from build123d import *

# Parameters (mm, degrees)
F0_W      = 46
F0_H      = 40
F1_DEPTH  = 46
F2_R      = 9
F3_DEPTH  = 30
F4_R      = 9
F5_DEPTH  = 30
F6_W      = 24
F6_H      = 30
F7_DEPTH  = 46
F9_R      = 18
F10_DEPTH = 25
F8_R      = 9
F11_DEPTH = 30
F12_R     = 18
F13_DEPTH = 30
F14_R     = 9
F15_DEPTH = 30


with BuildPart() as f1:
    # F0 (on Top) → F1 (new body)
    with BuildSketch(Plane.XY):
        with Locations((-30.6679215729, -38.7895996869)):
            Rectangle(F0_W, F0_H)
    extrude(amount=F1_DEPTH)

    # F2 (on face) → F3 (join)
    with BuildSketch(Plane(origin=(-53.6679215729, 0, 0), x_dir=(0, -1, 0), z_dir=(-1, 0, 0))):
        with Locations((35.7066951692, 22.7147787809)):
            Circle(F2_R)
    extrude(amount=F3_DEPTH)

    # F4 (on face) → F5 (join)
    with BuildSketch(Plane.YZ.offset(-7.6679215729)):
        with Locations((-38.5694056749, 23.5416200012)):
            Circle(F4_R)
    extrude(amount=F5_DEPTH)

    # F6 (on face) → F7 (cut)
    with BuildSketch(Plane.XZ.offset(58.7895996869)):
        with Locations((-28.5605824441, 23.7626548484)):
            Rectangle(F6_W, F6_H)
    extrude(amount=-F7_DEPTH, mode=Mode.SUBTRACT)

    # F9 (on face) → F10 (join)
    with BuildSketch(Plane(origin=(-53.6679215729, 0, 0), x_dir=(0, -1, 0), z_dir=(-1, 0, 0))):
        with Locations((35.7066951692, 22.7147787809)):
            Circle(F9_R)
    extrude(amount=F10_DEPTH)

    # F8 (on face) → F11 (cut)
    with BuildSketch(Plane(origin=(-83.6679215729, 0, 0), x_dir=(0, -1, 0), z_dir=(-1, 0, 0))):
        with Locations((35.7066951692, 22.7147787809)):
            Circle(F8_R)
    extrude(amount=-F11_DEPTH, mode=Mode.SUBTRACT)

    # F12 (on face) → F13 (join)
    with BuildSketch(Plane.YZ.offset(-7.6679215729)):
        with Locations((-38.5694056749, 23.5416200012)):
            Circle(F12_R)
    extrude(amount=F13_DEPTH)

    # F14 (on face) → F15 (cut)
    with BuildSketch(Plane.YZ.offset(22.3320784271)):
        with Locations((-38.5694056749, 23.5416200012)):
            Circle(F14_R)
    extrude(amount=-F15_DEPTH, mode=Mode.SUBTRACT)


solid = f1.part
Input: part model. Units: mm. Frame: model coordinates. A direction names the side the tool comes from. Give positions to 0.01 mm unless a question says otherwise; leave off trailing zeros. Write each loop counter-clockwise with the first axis right and the second up, starting at its lowest first coordinate (ties: lowest second). Pieces come first, ordered by that corner, then holes.
Q1. First-contact query: P1, Ø14, axis at x = -32.5, z = 34, coming from the +Y side; P2, Ø3, axis at x = -62.5, z = 23, coming from the -Y side; P3, Ø0.5, axis at y = -18, z = 23, coming from the +X side. Flat tips, straight axial feed; report the tip coordinate or a pass-through.
Q2. Pull-direction query (X, two-part tool) for faces 5 (the face through (-53.668, -36, 23)), 6 (the face through (-40.561, -39, 24)), 7 (the face through (-65.993, -52.875, 28.121)); classes: pulls with the +X half, pulls with the -X half, needs draft (parallel to the pull), parting line crosses it, or undercut.
Q3. Section D-D, the plane y = -49.5. Output: boundary loops of the cut face in (x, z), plus the area to 3 significant figures.
Q4. Section A-A, the plane y = -40.5. Output: boundary loops of the cut face in (x, z).
Q5. Section B-B, the plane z = 30.5. Output: boundary loops of the cut face in (x, y), plus the area to 3 significant figures.
Q6. Material intervals for probe 1 along X at (y, z) = (-55, 38.5); probe 2 along Z at (x, y) = (-19.5, -19); probe 3 along X at (y, z) = (-48, 16), sorted ascending.
Q7. Set-up query: faces 1 (the face through (7.122, -52.854, 12.589)), 2 (the face through (-16.561, -39, 24)), 3 (the face through (-66.343, -29.073, 28.797)), 4 (the face through (-41, -18.79, 23)). Return all of +Z, -Z, +X, -X, +Y, -Y with unobstructed straight access to the full face (end or side cutting, diameter ignored); none if empty.
Q8. Section C-C, the plane x = -45.5. Output: boundary loops of the cut face in (y, z).
Filled in:
1. P1: stops at y = -18.79
1. P2: stops at y = -53.71
1. P3: stops at x = -53.67
2. face 5: pulls with the -X half
2. face 6: undercut
2. face 7: needs draft
3. outline: (-78.67, 11.15) - (-53.67, 11.15) - (-53.67, 0) - (-7.67, 0) - (-7.67, 9.24) - (22.33, 9.24) - (22.33, 37.84) - (-7.67, 37.84) - (-7.67, 46) - (-53.67, 46) - (-53.67, 34.28) - (-78.67, 34.28) - close; hole (-40.56, 8.76) - (-16.56, 8.76) - (-16.56, 38.76) - (-40.56, 38.76) - close
3. area: 2,830 mm2
4. outline: (-78.67, 5.36) - (-53.67, 5.36) - (-53.67, 0) - (-7.67, 0) - (-7.67, 5.65) - (22.33, 5.65) - (22.33, 14.75) - (-7.67, 14.75) - (-7.67, 32.33) - (22.33, 32.33) - (22.33, 41.44) - (-7.67, 41.44) - (-7.67, 46) - (-53.67, 46) - (-53.67, 40.06) - (-78.67, 40.06) - (-78.67, 30.33) - (-53.67, 30.33) - (-53.67, 15.1) - (-78.67, 15.1) - close; hole (-40.56, 8.76) - (-16.56, 8.76) - (-16.56, 38.76) - (-40.56, 38.76) - close
5. outline: (-78.67, -51.94) - (-53.67, -51.94) - (-53.67, -58.79) - (-40.56, -58.79) - (-40.56, -18.79) - (-53.67, -18.79) - (-53.67, -19.48) - (-78.67, -19.48) - (-78.67, -31.19) - (-53.67, -31.19) - (-53.67, -40.22) - (-78.67, -40.22) - close; (-16.56, -58.79) - (-7.67, -58.79) - (-7.67, -55.17) - (22.33, -55.17) - (22.33, -44.28) - (-7.67, -44.28) - (-7.67, -32.86) - (22.33, -32.86) - (22.33, -21.97) - (-7.67, -21.97) - (-7.67, -18.79) - (-16.56, -18.79) - close
5. area: 2,120 mm2
6. probe 1: x = -53.67 to -40.56, -16.56 to -7.67
6. probe 2: z = 0 to 8.76, 38.76 to 46
6. probe 3: x = -78.67 to -40.56, -16.56 to 22.33
7. face 1: +X
7. face 2: +Y, -Y
7. face 3: -X
7. face 4: +Z, -Z, +X, +Y
8. outline: (-58.79, 0) - (-18.79, 0) - (-18.79, 46) - (-58.79, 46) - close
